Input: part model. Units: mm. Frame: model coordinates. Face numbers are marked on the shaded views. A direction names the side the tool comes from. Give positions to 0.01 mm unless a question says otherwise; leave off trailing zeros. Order: outer loops, then holes, each group sorted by start corner. A loop starts at its lowest first (then second) coordinate and runs counter-clockwise, first axis right, second up. Notation, with made-up numbers: (36, -0.5) - (43, -0.5) arc R19 cw to (43, 20.5) - close; hole circle Ø6 at (26.5, 23). An arc over 180 degrees is marked (long way). Answer in a Markdown table with one row per item. Add a question column.
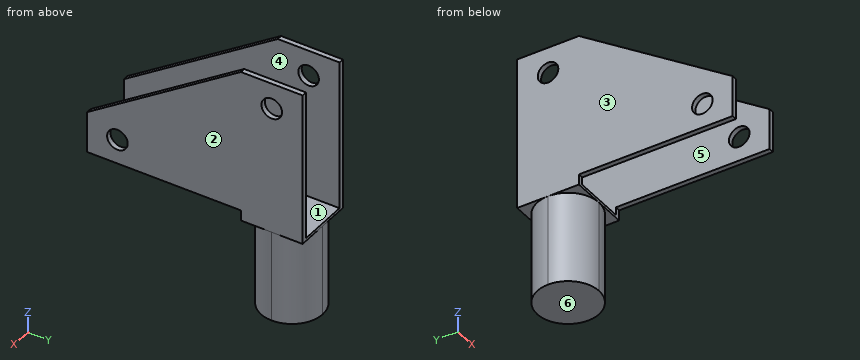
from build123d import *

# Parameters (mm, degrees)
F0_R          = 2
F1_DEPTH      = 6
F2_W          = 10
F2_H          = 33.9879472775
F3_DEPTH      = 6.001
F3_DEPTH_BACK = 35.8828483539
F5_DEPTH      = 17.7


with BuildPart() as f1:
    # F0 (on Right) → F1 (new body, symmetric)
    with BuildSketch(Plane.YZ):
        Polygon((-6, 4.9863578752), (-35.8818483539, -14.7544573992), (-35.8818483539, -22.7532479912), (-6, -22.7532479912), (-6, -42.48220101), (6, -42.48220101), (6, 4.9863578752), align=None)
        with Locations((-30, -18)):
            Circle(F0_R, mode=Mode.SUBTRACT)
        Circle(F0_R, mode=Mode.SUBTRACT)
    extrude(amount=F1_DEPTH, both=True)

    # F2 (on Front) → F3 (cut, two sides)
    with BuildSketch(Plane.XZ) as f3_sk:
        with Locations((0, -7.2282501862)):
            Rectangle(F2_W, F2_H)
    extrude(amount=-F3_DEPTH, mode=Mode.SUBTRACT)
    extrude(f3_sk.sketch, amount=F3_DEPTH_BACK, mode=Mode.SUBTRACT)

    # F4 (on face) → F5 (cut)
    with BuildSketch(Plane(origin=(0, 0, -42.48220101), x_dir=(1, 0, 0), z_dir=(0, 0, -1))):
        with BuildLine():
            Line((-6, -6), (0, -6))
            ThreePointArc((0, -6), (-4.2426406871, -4.2426406871), (-6, 0))
            Line((-6, 0), (-6, -6))
        make_face()
        with BuildLine():
            ThreePointArc((-6, 0), (-4.2426406871, 4.2426406871), (0, 6))
            Line((0, 6), (-6, 6))
            Line((-6, 6), (-6, 0))
        make_face()
        with BuildLine():
            ThreePointArc((0, 6), (4.2426406871, 4.2426406871), (6, 0))
            Line((6, 0), (6, 6))
            Line((6, 6), (0, 6))
        make_face()
        with BuildLine():
            Line((6, -6), (6, 0))
            ThreePointArc((6, 0), (4.2426406871, -4.2426406871), (0, -6))
            Line((0, -6), (6, -6))
        make_face()
    extrude(amount=-F5_DEPTH, mode=Mode.SUBTRACT)


solid = f1.part
Q1. Line query: probe 1 along X at (y, z) = (-0.5, -6.5); probe 2 along Z at (x, y) = (5.65, 0); probe 3 along Z at (x, y) = (0.75, -4). Output: solid intervals per line, ascending.
Q2. Contact query for flat-ended pins moving along their axis: P1, Ø5, axis at x = 1.5, z = -32, coming from the +Y side; P2, Ø6, axis at x = 4.5, z = -4.5, coming from the -Y side; P3, Ø6, axis at x = -1.5, z = -37, coming from the -Y side; P4, Ø0.5, axis at x = -5.5, y = -17.5, coming from the -Z side. Output: stop coordinate, or through.
Q3. Pull-direction query (X, two-part tool) for the marked faces 1, 2, 3 and 4; classes: +X half, -X half, draft (parallel to the pull), parting line (faces both ways), or undercut.
Q4. Section D-D, the plane x = 2. Return loops of the section in (y, z), then the cut area to 3 significant figures.
Q5. Section B-B, the plane y = -27. Return loops of the section in (x, z).
Q6. Section A-A, the plane z = -18. Return loops of the section in (x, y).
Q7. Section C-C, the plane z = -9. Return loops of the section in (x, y).
Q8. Access query for the marked faces 5 and 6. Directions: +Z, -Z, +X, -X, +Y, -Y. A direction counts if a zero-diameter tool reaches every point of the face in a straight line with its end or side. Return the directions, or none.
Computed:
| question | item | result |
|---|---|---|
| 1 | probe 1 | x = -6 to -5, 5 to 6 |
| 1 | probe 2 | z = -42.48 to -2, 2 to 4.99 |
| 1 | probe 3 | z = -42.48 to -24.22 |
| 2 | P1 | stops at y = 6 |
| 2 | P2 | stops at y = -24.84 |
| 2 | P3 | stops at y = -6 |
| 2 | P4 | stops at z = -22.75 |
| 3 | face 1 | undercut |
| 3 | face 2 | +X half |
| 3 | face 3 | -X half |
| 3 | face 4 | undercut |
| 4 | outline | (-6, -24.78) - (-5.66, -24.78) - (-5.66, -42.48) - (5.66, -42.48) - (5.66, -24.78) - (6, -24.78) - (6, -24.22) - (-6, -24.22) - close |
| 4 | area | 207 mm^2 |
| 5 | outline | (-6, -22.75) - (-5, -22.75) - (-5, -8.89) - (-6, -8.89) - close; (5, -22.75) - (6, -22.75) - (6, -8.89) - (5, -8.89) - close |
| 6 | outline | (-6, -35.88) - (-5, -35.88) - (-5, -32) - (-6, -32) - close; (-6, -28) - (-5, -28) - (-5, 6) - (-6, 6) - close; (5, -35.88) - (6, -35.88) - (6, -32) - (5, -32) - close; (5, -28) - (6, -28) - (6, 6) - (5, 6) - close |
| 7 | outline | (-6, -27.17) - (-5, -27.17) - (-5, 6) - (-6, 6) - close; (5, -27.17) - (6, -27.17) - (6, 6) - (5, 6) - close |
| 8 | face 5 | +Z, +Y, -Y |
| 8 | face 6 | -Z, +X, -X, +Y, -Y |
